Verification items for the finished model (mm, model axes). Face numbers are marked on the shaded views. A direction names the side the tool comes from. Round coordinates to 2 decimals unless told otherwise and drop trailing zeros. Loops run counter-clockwise (first coordinate to the right, second up) from the corner with the lowest first, then second, coordinate; pieces in that order, holes last. Notation, with made-up numbers: (74.25, 20) - (128.25, 20) arc R30 ccw to (128.25, 52) - close; hole circle Ø2 at (-16, 32). An arc over 180 degrees is marked (long way). Use a Markdown table: item, result. Add a question column.
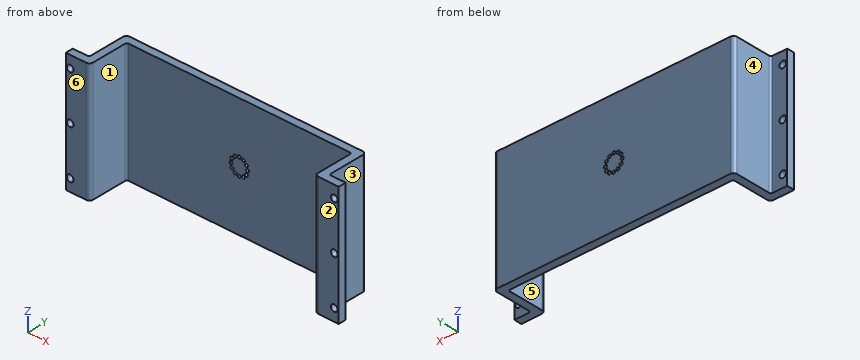
```python
from build123d import *

# Parameters (mm, degrees)
BOSS_EXTRUDE1_DEPTH            = 100
FILLET1_R                      = 3
FILLET1_2_R                    = 1.5
F_2_5MM_DOWEL_HOLE1_AT_2_COUNT = 2
F_2_5MM_DOWEL_HOLE1_AT_2_PITCH = 14
CIRPATTERN3_COUNT              = 6
CIRPATTERN3_ANGLE              = 150
F_5_5_5_5_DIAMETER_HOLE1_D     = 5.5


with BuildPart() as part:
    # Sketch1 → Boss-Extrude1 (new body)
    with BuildSketch(Plane.XY):
        Polygon((100, 0), (-100, 0), (-100, -33.65), (-113.65, -33.65), (-113.65, -40), (-93.65, -40), (-93.65, -6.35), (93.65, -6.35), (93.65, -40), (113.65, -40), (113.65, -33.65), (100, -33.65), align=None)
    extrude(amount=BOSS_EXTRUDE1_DEPTH)

    # Fillet1
    fillet1_edges = [part.edges().sort_by_distance(p)[0] for p in [
        (-100, 0, 50),
        (-93.65, -40, 50),
        (100, 0, 50),
        (93.65, -40, 50),
    ]]
    fillet(fillet1_edges, radius=FILLET1_R)

    # Fillet1 2
    fillet1_2_edges = [part.edges().sort_by_distance(p)[0] for p in [
        (-93.65, -6.35, 50),
        (93.65, -6.35, 50),
        (100, -33.65, 50),
        (-100, -33.65, 50),
    ]]
    fillet(fillet1_2_edges, radius=FILLET1_2_R)

    # Sketch2 → 2.5mm Dowel Hole1 (revolve, cut)
    with BuildSketch(Plane(origin=(0, -6.35, 57), x_dir=(0, 0, -1), z_dir=(1, 0, 0))):
        Polygon((0, 0), (0, 10.751075774), (1.25, 10), (1.25, 0), align=None)
    f_2_5mm_dowel_hole1 = revolve(axis=Axis((0, -12.7, 57), (0, 1, 0)), mode=Mode.SUBTRACT)

    # 2.5mm Dowel Hole1 at 2: 2.5mm Dowel Hole1 ×2
    with Locations(*[(0, 0, -i * F_2_5MM_DOWEL_HOLE1_AT_2_PITCH) for i in range(1, F_2_5MM_DOWEL_HOLE1_AT_2_COUNT)]):
        add(f_2_5mm_dowel_hole1, mode=Mode.SUBTRACT)

    # CirPattern3: 2.5mm Dowel Hole1 ×6 about axis
    cirpattern3_axis = Axis((0, 0, 50), (0, -1, 0))
    for i in range(1, CIRPATTERN3_COUNT):
        add(f_2_5mm_dowel_hole1.rotate(cirpattern3_axis, i * CIRPATTERN3_ANGLE / (CIRPATTERN3_COUNT - 1)), mode=Mode.SUBTRACT)

    # CirPattern3 copy 1 sketch → CirPattern3 copy 1 (revolve, cut)
    with BuildSketch(Plane(origin=(3.5, -6.35, 43.937822174), x_dir=(0.5, 0, -0.866025404), z_dir=(0.866025404, 0, 0.5))):
        Polygon((0, 0), (0, 10.751075774), (1.25, 10), (1.25, 0), align=None)
    revolve(axis=Axis((3.5, -12.7, 43.937822174), (0, 1, 0)), mode=Mode.SUBTRACT)

    # CirPattern3 copy 2 sketch → CirPattern3 copy 2 (revolve, cut)
    with BuildSketch(Plane(origin=(6.062177826, -6.35, 46.5), x_dir=(0.866025404, 0, -0.5), z_dir=(0.5, 0, 0.866025404))):
        Polygon((0, 0), (0, 10.751075774), (1.25, 10), (1.25, 0), align=None)
    revolve(axis=Axis((6.062177826, -12.7, 46.5), (0, 1, 0)), mode=Mode.SUBTRACT)

    # CirPattern3 copy 3 sketch → CirPattern3 copy 3 (revolve, cut)
    with BuildSketch(Plane(origin=(7, -6.35, 50), x_dir=(1, 0, 0), z_dir=(0, 0, 1))):
        Polygon((0, 0), (0, 10.751075774), (1.25, 10), (1.25, 0), align=None)
    revolve(axis=Axis((7, -12.7, 50), (0, 1, 0)), mode=Mode.SUBTRACT)

    # CirPattern3 copy 4 sketch → CirPattern3 copy 4 (revolve, cut)
    with BuildSketch(Plane(origin=(6.062177826, -6.35, 53.5), x_dir=(0.866025404, 0, 0.5), z_dir=(-0.5, 0, 0.866025404))):
        Polygon((0, 0), (0, 10.751075774), (1.25, 10), (1.25, 0), align=None)
    revolve(axis=Axis((6.062177826, -12.7, 53.5), (0, 1, 0)), mode=Mode.SUBTRACT)

    # CirPattern3 copy 5 sketch → CirPattern3 copy 5 (revolve, cut)
    with BuildSketch(Plane(origin=(3.5, -6.35, 56.062177826), x_dir=(0.5, 0, 0.866025404), z_dir=(-0.866025404, 0, 0.5))):
        Polygon((0, 0), (0, 10.751075774), (1.25, 10), (1.25, 0), align=None)
    revolve(axis=Axis((3.5, -12.7, 56.062177826), (0, 1, 0)), mode=Mode.SUBTRACT)

    # 5.5 _5.5_ Diameter Hole1 (through all)
    with Locations(Plane(origin=(0, -33.65, 0), x_dir=(1, 0, 0), z_dir=(0, 1, 0))):
        with Locations((-110, -10), (-110, -50), (-110, -90), (110, -90), (110, -50), (110, -10)):
            Hole(F_5_5_5_5_DIAMETER_HOLE1_D / 2)


solid = part.part
```
Q1. Thickness scan on line 1 along Z through (x, y) = (3.5, -3.25); line 2 along Z through (x, y) = (0, -4.5); line 3 along X through (y, z) = (-36, 10). Record the ranges inside material, lowest first.
Q2. Section check C-C on x = 38. Record the cut outline in (y, z).
Q3. Go/stop test with flat-tipped pins: pin 1 Ø3 at (x, z) = (-3.5, 43.94) entering from -Y; pin 2 Ø8 at (y, z) = (-12, 29) entering from +X; pin 3 Ø3 at (x, z) = (0, 43) entering from +Y; pin 4 Ø6.5 at (x, z) = (-110, 10) entering from +Y. Record where each tip stops, or that it passes through.
Q4. Set-up check for the marked faces 4, 5 and 6: record each of +Z, -Z, +X, -X, +Y, -Y from which the full face is reachable in a straight line by a thin tool's end or side.
Q5. Section check B-B on y = -24.5. Record the cut outline in (x, z).
Q6. Release check for a two-part mould opening along X. For the marked faces 1, 2 and 3 record: +X half, -X half, draft (parallel to the pull), parting line (faces both ways), or undercut.
Q7. Section check A-A on z = 10. Record the cut outline in (x, y).
Determined:
| question | item | result |
|---|---|---|
| 1 | line 1 | z = 0 to 42.69, 45.19 to 54.81, 57.31 to 100 |
| 1 | line 2 | z = 0 to 41.75, 44.25 to 55.75, 58.25 to 100 |
| 1 | line 3 | x = -113.65 to -112.75, -107.25 to -93.65, 93.65 to 107.25, 112.75 to 113.65 |
| 2 | outline | (-6.35, 0) - (0, 0) - (0, 100) - (-6.35, 100) - close |
| 3 | pin 1 | stops at y = -6.35 |
| 3 | pin 2 | stops at x = 100 |
| 3 | pin 3 | stops at y = 0 |
| 3 | pin 4 | stops at y = -33.65 |
| 4 | face 4 | +Z, -Z, -X, +Y |
| 4 | face 5 | +Z, -Z, -Y |
| 4 | face 6 | +Z, -Z, +X, -X, -Y |
| 5 | outline | (-100, 0) - (-93.65, 0) - (-93.65, 100) - (-100, 100) - close; (93.65, 0) - (100, 0) - (100, 100) - (93.65, 100) - close |
| 6 | face 1 | undercut |
| 6 | face 2 | draft |
| 6 | face 3 | +X half |
| 7 | outline | (-113.65, -40) - (-112.75, -40) - (-112.75, -33.65) - (-113.65, -33.65) - close; (-107.25, -40) - (-96.65, -40) arc R3 ccw to (-93.65, -37) - (-93.65, -7.85) arc R1.5 cw to (-92.15, -6.35) - (92.15, -6.35) arc R1.5 cw to (93.65, -7.85) - (93.65, -37) arc R3 ccw to (96.65, -40) - (107.25, -40) - (107.25, -33.65) - (101.5, -33.65) arc R1.5 cw to (100, -32.15) - (100, -3) arc R3 ccw to (97, 0) - (-97, 0) arc R3 ccw to (-100, -3) - (-100, -32.15) arc R1.5 cw to (-101.5, -33.65) - (-107.25, -33.65) - close; (112.75, -40) - (113.65, -40) - (113.65, -33.65) - (112.75, -33.65) - close |
